Check sheet for the modelled part. Datum: model origin and axes. Units: mm. Face numbers are marked on the shaded views. Round coordinates to 2 decimals unless told otherwise and drop trailing zeros. Order: outer loops, then holes, each group sorted by start corner. A loop starts at its lowest first (then second) coordinate and runs counter-clockwise, first axis right, second up.
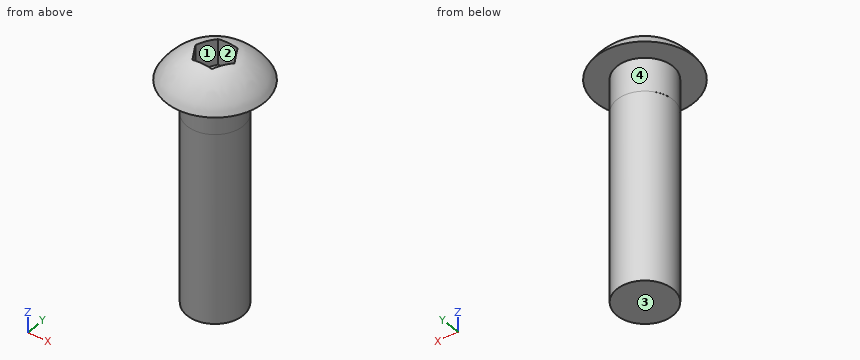
Solid Edge part; units mm, degrees
sketch "Sketch1" plane through (0, 0, 0) normal (1, 0, 0) x (0, 1, 0)
  line L0 (0, -2.1082) -> (0, 2.1082)
  arc A0 (0, 2.1082) -> (6.9469, -2.1082) centre (-0.3606, -6.3169) cw
  line L1 (0, -2.1082) -> (6.9469, -2.1082)
revolve "RevolvedProtrusion1" add sketch "Sketch1" angle 360 about axis through (0, 0, -14.7796) along (0, 0, 1)
sketch "Sketch2" plane through (0, 0, -2.1082) normal (0, 0, -1) x (0, 1, 0)
  circle A0 centre (0, 0) radius 3.9687
extrude "Protrusion1" add sketch "Sketch2" along normal blind 31.75
sketch "Sketch3" plane through (0, 0, -33.8582) normal (0, 0, -1) x (1, 0, 0)
  circle A0 centre (0, 0) radius 3.9662
extrude "Cutout1" cut sketch "Sketch3" against normal blind 27.0002 flip side to cut
sketch "Sketch4" plane through (-0.6032, 0.3606, 4.2164) normal (0, 0, 1) x (1, 0, 0)
  line L0 (-0.7716, 2.0206) -> (1.978, 2.0206)
  line L1 (3.3529, -0.3606) -> (1.978, 2.0206)
  line L2 (1.978, -2.7419) -> (3.3529, -0.3606)
  line L3 (-0.7716, -2.7419) -> (1.978, -2.7419)
  line L4 (-2.1464, -0.3606) -> (-0.7716, -2.7419)
  line L5 (-0.7716, 2.0206) -> (-2.1464, -0.3606)
extrude "ExtrudedCutout_11" cut sketch "Sketch4" against normal blind 6.3246
properties part number "209090"
Item 1: Sectioned sample at A-A (z = -14). Record the cut outline in (x, y).
Answer:
outline: circle Ø7.93 at (0, 0)
Item 2: Scan lines: line 1 along Z through (x, y) = (-1.25, 4.5); line 2 along Y through (x, z) = (1.75, -4); line 3 along X through (y, z) = (-3.5, -31). Record each from-to range of solid material in increasing order.
Answer:
line 1: z = -2.11 to 0.45
line 2: y = -3.56 to 3.56
line 3: x = -1.87 to 1.87
Item 3: Release check for a two-part mould opening along X. For the marked faces 1, 2, 3 and 4 record: released by +X, released by -X, zero draft, split by the parting line, or undercut.
Answer:
face 1: undercut
face 2: undercut
face 3: zero draft
face 4: split by the parting line
Item 4: Go/stop test with flat-tipped pins: P1, Ø2.5, axis at x = 0.5, y = 0, coming from the +Z side; P2, Ø8, axis at y = -4, z = -15.5, coming from the -X side; P3, Ø6, axis at x = -1, z = -13.5, coming from the -Y side. Record where each tip stops, or that it passes through.
Answer:
P1: stops at z = -2.11
P2: stops at x = -3.97
P3: stops at y = -3.97
